Work out the finished part from the listing and answer in its coordinate system (mm). Face numbers are marked on the shaded views. Round coordinates to 2 decimals unless told otherwise and drop trailing zeros. Order: outer loops, then holes, each group sorted by start corner. A loop starts at its lowest first (then second) coordinate and runs counter-clockwise, first axis right, second up. Notation, with made-up numbers: (-36.75, -2) - (-20.75, -2) arc R21 cw to (-20.75, 16) - close; hole circle Ø3 at (70, -3.5). An arc over 180 degrees is marked (long way). Answer in a Markdown table with one row per item.
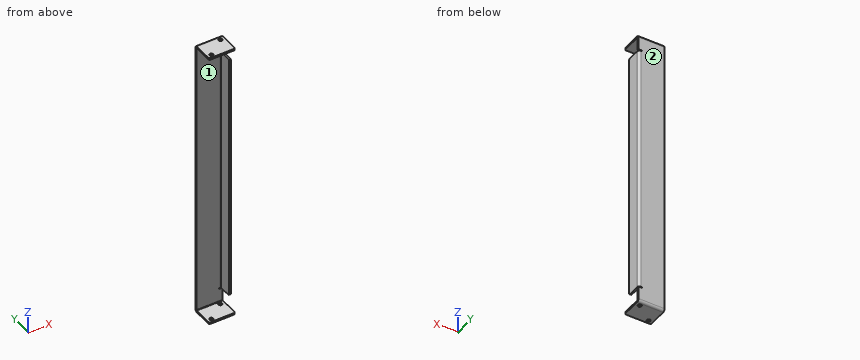
from build123d import *

# Parameters (mm, degrees)
SKETCH1_W                    = 327
SKETCH1_H                    = 2
BASE_FLANGE1_DEPTH           = 15
EDGE_FLANGE1_STRIP_W         = 9.4732
EDGE_FLANGE1_STRIP_H         = 2
EDGE_FLANGE1_STRIP_CUT_DEPTH = 30
EDGE_FLANGE1_DEPTH           = 30
CUT_EXTRUDE1_REACH           = 329.582
SKETCH9_R                    = 2.1
EDGE_FLANGE2_START           = 9.7634
EDGE_FLANGE2_DEPTH           = 3.2366
EDGE_FLANGE2_START_2         = -4.5
EDGE_FLANGE2_2_OUTLINE_W     = 2
EDGE_FLANGE2_2_OUTLINE_H     = 290
EDGE_FLANGE2_2_DEPTH         = 14.2634
EDGE_FLANGE2_START_3         = -145
EDGE_FLANGE2_3_DEPTH         = 290
EDGE_FLANGE2_4_DEPTH         = 290
FILLET1_R                    = 1.5


with BuildPart() as part:
    # Base-Flange1: sheet metal written as solids
    # Sketch1 → Base-Flange1 (new, symmetric)
    with BuildSketch(Plane(origin=(0, 0, 0), x_dir=(0, 0, -1), z_dir=(1, 0, 0))):
        with Locations((0, 11.5)):
            Rectangle(SKETCH1_W, SKETCH1_H)
    extrude(amount=BASE_FLANGE1_DEPTH, both=True)

    # Edge-Flange1: sheet metal written as solids
    # Edge-Flange1 strip (on a plane across the edge) → Edge-Flange1 strip cut (cut)
    with BuildSketch(Plane(origin=(15, 10.5, 163.5), x_dir=(0, 0, -1), z_dir=(-1, 0, 0))):
        with Locations((-2, -1)):
            Rectangle(EDGE_FLANGE1_STRIP_W, EDGE_FLANGE1_STRIP_H)
    edge_flange1_strip_cut = extrude(amount=EDGE_FLANGE1_STRIP_CUT_DEPTH, mode=Mode.SUBTRACT)

    # Edge-Flange1 section (on a plane across the edge) → Edge-Flange1 (add)
    with BuildSketch(Plane(origin=(15, 10.5, 163.5), x_dir=(0, 0, -1), z_dir=(-1, 0, 0))):
        with BuildLine():
            Line((0, 0.7366), (0, 23))
            Line((0, 23), (2, 23))
            Line((2, 23), (2, 0.7366))
            ThreePointArc((2, 0.7366), (2.215745145, 0.215745145), (2.7366, 0))
            Line((2.7366, 0), (2.7366, -2))
            ThreePointArc((2.7366, -2), (0.801531583, -1.198468417), (0, 0.7366))
        make_face()
    edge_flange1 = extrude(amount=EDGE_FLANGE1_DEPTH)

    # Mirror1: Edge-Flange1 strip cut, Edge-Flange1 across plane
    add(edge_flange1_strip_cut.mirror(Plane.XY), mode=Mode.SUBTRACT)
    add(edge_flange1.mirror(Plane.XY))

    # Sketch9 → Cut-Extrude1 (cut, up to next)
    with BuildSketch(Plane.XY.offset(163.5), mode=Mode.PRIVATE) as cut_extrude1_sk1:
        with Locations((10, 6.666666667)):
            Circle(SKETCH9_R)
    cut_extrude1_tool1 = extrude(cut_extrude1_sk1.sketch, amount=-CUT_EXTRUDE1_REACH, mode=Mode.PRIVATE) & part.part
    # Sketch9 → Cut-Extrude1 (cut, up to next)
    with BuildSketch(Plane.XY.offset(163.5), mode=Mode.PRIVATE) as cut_extrude1_sk2:
        with Locations((-10, -8.666666667)):
            Circle(SKETCH9_R)
    cut_extrude1_tool2 = extrude(cut_extrude1_sk2.sketch, amount=-CUT_EXTRUDE1_REACH, mode=Mode.PRIVATE) & part.part
    cut_extrude1_1 = cut_extrude1_tool1.solids().sort_by_distance((10, 6.666667, 163.5))[0]
    add(cut_extrude1_1, mode=Mode.SUBTRACT)
    cut_extrude1_2 = cut_extrude1_tool2.solids().sort_by_distance((-10, -8.666667, 163.5))[0]
    add(cut_extrude1_2, mode=Mode.SUBTRACT)
    cut_extrude1 = cut_extrude1_1 + cut_extrude1_2  # Cut-Extrude1 as one shape, for the pattern or mirror that repeats it

    # Mirror2: Cut-Extrude1 across plane
    add(cut_extrude1.mirror(Plane.XY), mode=Mode.SUBTRACT)

    # Edge-Flange2: read off the stored shape, not the designer's step
    # Edge-Flange2 outline → Edge-Flange2 (cut)
    with BuildSketch(Plane(origin=(0, 0, 0), x_dir=(1, 0, 0), z_dir=(0, 1, 0)).offset(EDGE_FLANGE2_START)):
        with BuildLine():
            Line((15, -146), (15, -145))
            Line((15, -145), (11.2634, -145))
            ThreePointArc((11.2634, -145), (10.7634, -145.5), (11.2634, -146))
            Line((11.2634, -146), (15, -146))
        make_face()
        with BuildLine():
            Line((11.2634, 145), (15, 145))
            Line((15, 145), (15, 146))
            Line((15, 146), (11.2634, 146))
            ThreePointArc((11.2634, 146), (10.7634, 145.5), (11.2634, 145))
        make_face()
    extrude(amount=EDGE_FLANGE2_DEPTH, mode=Mode.SUBTRACT)

    # Edge-Flange2 3 outline → Edge-Flange2 3 (cut)
    with BuildSketch(Plane.XY.offset(EDGE_FLANGE2_START_3)):
        with BuildLine():
            ThreePointArc((12.2634, 12.5), (13.917667209, 11.943395312), (14.899002398, 10.5))
            Line((14.899002398, 10.5), (15, 10.5))
            Line((15, 10.5), (15, 12.5))
            Line((15, 12.5), (12.2634, 12.5))
        make_face()
    extrude(amount=EDGE_FLANGE2_3_DEPTH, mode=Mode.SUBTRACT)



with BuildPart() as body_2:
    # Edge-Flange2 2 outline → Edge-Flange2 2 (new body)
    with BuildSketch(Plane(origin=(0, 0, 0), x_dir=(1, 0, 0), z_dir=(0, 1, 0)).offset(EDGE_FLANGE2_START_2)):
        with Locations((14, 0)):
            Rectangle(EDGE_FLANGE2_2_OUTLINE_W, EDGE_FLANGE2_2_OUTLINE_H)
    extrude(amount=EDGE_FLANGE2_2_DEPTH)


with BuildPart() as part_1:
    add(part.part)

    add(body_2.part)  # Edge-Flange2 4 merges body 2
    # Edge-Flange2 4 outline → Edge-Flange2 4 (add)
    with BuildSketch(Plane.XY.offset(EDGE_FLANGE2_START_3)):
        with BuildLine():
            Line((13, 9.7634), (15, 9.7634))
            ThreePointArc((15, 9.7634), (14.974633029, 10.135145906), (14.899002398, 10.5))
            Line((14.899002398, 10.5), (12.2634, 10.5))
            ThreePointArc((12.2634, 10.5), (12.784254855, 10.284254855), (13, 9.7634))
        make_face()
    extrude(amount=EDGE_FLANGE2_4_DEPTH)

    # Fillet1
    fillet1_edges = [part_1.edges().sort_by_distance(p)[0] for p in [
        (15, 11.5, 146),
        (15, 11.5, -146),
        (14, -4.5, -145),
        (14, -4.5, 145),
        (15, -12.5, 162.5),
        (-15, -12.5, 162.5),
        (-15, -12.5, -162.5),
        (15, -12.5, -162.5),
    ]]
    fillet(fillet1_edges, radius=FILLET1_R)


solid = part_1.part
1) Find section B-B, the plane z = -56. Give the vertices of the cut face in (x, y).
Filled in:
| item | result |
|---|---|
| outline | (-15, 10.5) - (12.26, 10.5) arc R0.74 cw to (13, 9.76) - (13, -4.5) - (15, -4.5) - (15, 9.76) arc R2.74 ccw to (12.26, 12.5) - (-15, 12.5) - close |
2) Find the intervals of material crossed by probe 1 along Z at (x, y) = (-4.5, 5); probe 2 along X at (y, z) = (4.25, -41); probe 3 along Y at (x, z) = (-1, 72.5), in increasing order. Write a range as from..to.
Filled in:
| item | result |
|---|---|
| probe 1 | z = -163.5..-161.5, 161.5..163.5 |
| probe 2 | x = 13..15 |
| probe 3 | y = 10.5..12.5 |
3) The mould has two halves that part along Z. Classify the marked faces 1 and 2: released by +Z, released by -Z, zero draft, split by the parting line, or undercut.
Filled in:
| item | result |
|---|---|
| face 1 | undercut |
| face 2 | zero draft |
4) Find section A-A, the plane x = -2.5. Give the vertices of the cut face in (y, z).
Filled in:
| item | result |
|---|---|
| outline | (-12.5, -163.5) - (9.76, -163.5) arc R2.74 ccw to (12.5, -160.76) - (12.5, 160.76) arc R2.74 ccw to (9.76, 163.5) - (-12.5, 163.5) - (-12.5, 161.5) - (9.76, 161.5) arc R0.74 cw to (10.5, 160.76) - (10.5, -160.76) arc R0.74 cw to (9.76, -161.5) - (-12.5, -161.5) - close |
5) Each of these flat-tipped pins is pushed along its axis until it touches: pin 1 (1 mm diameter, centred on x = 12.5, y = 11.5, fed in from -Z); pin 2 (11.5 mm diameter, centred on y = 5, z = 18, fed in from -X); pin 3 (1 mm diameter, centred on x = 14, z = 61.5, fed in from -Y); pin 4 (8 mm diameter, centred on x = -9, z = 10.5, fed in from -Y). Where does it stop, or does it pass through?
Filled in:
| item | result |
|---|---|
| pin 1 | stops at z = -163.2 |
| pin 2 | stops at x = -15 |
| pin 3 | stops at y = -4.5 |
| pin 4 | stops at y = 10.5 |
